Model file for the job. Use its own axes, mm. A direction names the side the tool comes from. Round coordinates to 2 decimals unless told otherwise and drop trailing zeros. Order: outer loops, then holes, each group sorted by start corner. A loop starts at its lowest first (then second) coordinate and runs counter-clockwise, first axis right, second up. Notation, with made-up numbers: (13.5, -16.75) - (57.5, -16.75) arc R18 ccw to (57.5, 17.25) - close; hole circle Ø4 at (24.5, 21). An arc over 180 degrees is marked (long way). Use one line per item in the form item = value.
from build123d import *

# Parameters (mm, degrees)
F0_R      = 4
F1_DEPTH  = 28
F2_SIZE   = 0.1
F3_R      = 4
F4_DEPTH  = 6.5
F5_R      = 16.5
F6_DEPTH  = 4
F7_R      = 1
F8_DEPTH  = 4
F9_W      = 3
F9_H      = 1.5
F10_DEPTH = 15


with BuildPart() as f1:
    # F0 (on Front) → F1 (new body)
    with BuildSketch(Plane.XZ):
        Circle(F0_R)
    extrude(amount=-F1_DEPTH)

    # F2
    f2_edges = [f1.edges().sort_by_distance(p)[0] for p in [
        (-4, 0, 0),
    ]]
    chamfer(f2_edges, length=F2_SIZE)

    # F3 (on face) → F4 (join)
    with BuildSketch(Plane(origin=(0, 28, 0), x_dir=(-1, 0, 0), z_dir=(0, 1, 0))):
        Circle(F3_R)
    extrude(amount=F4_DEPTH)

    # F5 (on face) → F6 (join)
    with BuildSketch(Plane(origin=(0, 34.5, 0), x_dir=(-1, 0, 0), z_dir=(0, 1, 0))):
        Circle(F5_R)
    extrude(amount=F6_DEPTH)

    # F7 (on face) → F8 (join)
    with BuildSketch(Plane(origin=(0, 38.5, 0), x_dir=(-1, 0, 0), z_dir=(0, 1, 0))):
        with Locations((0, 13)):
            Circle(F7_R)
        with Locations((-13, 0)):
            Circle(F7_R)
        with Locations((0, -13)):
            Circle(F7_R)
        with Locations((13, 0)):
            Circle(F7_R)
    extrude(amount=F8_DEPTH)

    # F9 (on face) → F10 (cut)
    with BuildSketch(Plane.XZ):
        with Locations((0, 3.25)):
            Rectangle(F9_W, F9_H)
    extrude(amount=-F10_DEPTH, mode=Mode.SUBTRACT)


solid = f1.part
(1) Tool access for faces 5 (the face through (12, 40, 0)), 6 (the face through (-3, 34.5, -3)), 7 (the face through (-1.5, 7, 3)): list every direction of +Z, -Z, +X, -X, +Y, -Y with a clear straight run to the whole face (end or side of a thin tool).
Report:
face_5 = +Y
face_6 = -Y
face_7 = +Z, -Y
(2) Slice it at C-C on z = -13. Give the cut face in (x, y), then the cut area to 3 significant figures.
Report:
outline = (-10.16, 34.5) - (10.16, 34.5) - (10.16, 38.5) - (1, 38.5) - (1, 42.5) - (-1, 42.5) - (-1, 38.5) - (-10.16, 38.5) - close
area = 89.3 mm2
(3) Slice it at A-A on x = 0. Give the cut face in (y, z), then the cut area to 3 significant figures.
Report:
outline = (0, -3.9) - (0.1, -4) - (34.5, -4) - (34.5, -16.5) - (38.5, -16.5) - (38.5, -14) - (42.5, -14) - (42.5, -12) - (38.5, -12) - (38.5, 12) - (42.5, 12) - (42.5, 14) - (38.5, 14) - (38.5, 16.5) - (34.5, 16.5) - (34.5, 4) - (15, 4) - (15, 2.5) - (0, 2.5) - close
area = 401 mm2
(4) Pull direction X, two halves, no side cores. Call faces 1 (the face through (0, 7, 2.5)), 2 (the face through (0, 40, -14)), 3 (the face through (-14, 40, 0)), 4 (the face through (-13, 42.5, 0)): released by +X, released by -X, zero draft, split by the parting line, or undercut.
Report:
face_1 = undercut
face_2 = split by the parting line
face_3 = undercut
face_4 = zero draft
(5) Slice it at B-B on y = 9. Give the cut face in (x, z).
Report:
outline = (-1.5, 2.5) - (-1.5, 3.71) arc R4 ccw (long way) to (1.5, 3.71) - (1.5, 2.5) - close
(6) Pin check, flat tips, straight feed: pin 1 (3 mm diameter, centred on y = 30.5, z = -0.5, fed in from -X); pin 2 (10 mm diameter, centred on x = 10, z = -7, fed in from -Y); pin 3 (2 mm diameter, centred on y = 9.5, z = 2, fed in from +X). Stop position of each tip, or through.
Report:
pin_1 = -4
pin_2 = 34.5
pin_3 = 3.87
(7) Slice it at D-D on x = -13. Give the cut face in (y, z), then the cut area to 3 significant figures.
Report:
outline = (34.5, -10.16) - (38.5, -10.16) - (38.5, -1) - (42.5, -1) - (42.5, 1) - (38.5, 1) - (38.5, 10.16) - (34.5, 10.16) - close
area = 89.3 mm2
(8) Probe probe 1 along Y at (x, z) = (-6, -10); probe 2 along Z at (x, y) = (0, 17); probe 3 along Z at (x, y) = (3, 33). List the from-to ranges inside material, lowest first. Write a range as [from, to].
Report:
probe_1 = [34.5, 38.5]
probe_2 = [-4, 4]
probe_3 = [-2.65, 2.65]
